Could you check a few things on this model? Use its own coordinates, in mm. A direction names the side the tool comes from. Give positions to 0.01 mm unless a question says otherwise; leave off trailing zeros. Loops run counter-clockwise (first coordinate to the right, second up) from the corner with the lowest first, then second, coordinate; pieces in that order, holes last. Notation, with made-up numbers: (69, -3.5) - (101, -3.5) arc R29 ccw to (101, 21.5) - close; hole circle Ø7 at (13.25, -28.5). An arc over 180 degrees is marked (long way). One line per item, written item: value. Start each with the question number.
Q1. I want a section at C-C (x = 99). Please give me the cut outline in (y, z).
Q2. I want a section at A-A (x = -55). Please give me the cut outline in (y, z), then the cut area to 3 significant figures.
Q3. For faces 1 (the face through (67, -2.54, 18)), 2 (the face through (-51, -2.54, 188)), 3 (the face through (-69, 0, 18)), which set-ups out of +Z, -Z, +X, -X, +Y, -Y let a thin tool reach every point of the face, with its end or its side?
Q4. I'm going to push flat-ended pins straight in: P1, Ø6, axis at x = -57.5, z = 176.5, coming from the +Y side; P2, Ø0.8, axis at x = 85.5, y = -1, coming from the +Z side; P3, Ø10, axis at x = 92.5, z = -11.5, coming from the -Y side. Where does each tip first touch, or does it pass through?
Q5. I want a section at B-B (z = 82.5). Please give me the cut outline in (x, y) (3 decimals).
Q6. If I drill on line 1 (Z direction, x = -32.5, y = -1); line 2 (Y direction, x = -67.5, z = -40.5); line 3 (Y direction, x = -7.5, z = 166.5), over which ranges is the centre line in solid material (lowest first)? Write a range as from..to.
```python
from build123d import *

# Parameters (mm, degrees)
F0_W     = 9.525
F0_H     = 381
F2_W     = 184.15
F2_H     = 127
F2_W_2   = 254
F2_H_2   = 190.5
F3_DEPTH = 2.54


with BuildPart() as f1:
    # F0 (on Front) → F1 (revolve)
    with BuildSketch(Plane.XZ):
        with Locations((4.7625, 60.951888)):
            Rectangle(F0_W, F0_H)
    revolve(axis=Axis((0, 0, 60.951888), (0, 0, 1)))

    # F2 (on Front) → F3 (join)
    with BuildSketch(Plane.XZ):
        with Locations((0, 187.531114)):
            Rectangle(F2_W, F2_H)
        with Locations((0, 16.501888)):
            Rectangle(F2_W_2, F2_H_2)
    extrude(amount=F3_DEPTH)


solid = f1.part
```
Worked answers:
1. outline: (-2.54, -78.75) - (0, -78.75) - (0, 111.75) - (-2.54, 111.75) - close
2. outline: (-2.54, -78.75) - (0, -78.75) - (0, 111.75) - (-2.54, 111.75) - close; (-2.54, 124.03) - (0, 124.03) - (0, 251.03) - (-2.54, 251.03) - close
2. area: 806 mm²
3. face 1: +Z, -Z, +X, -Y
3. face 2: +Z, -Z, -X, -Y
3. face 3: +Z, -Z, -X, +Y
4. P1: stops at y = 0
4. P2: stops at z = 251.03
4. P3: stops at y = -2.54
5. outline: (-127, -2.54) - (-9.18, -2.54) arc R9.525 ccw to (9.18, -2.54) - (127, -2.54) - (127, 0) - (9.525, 0) arc R9.525 ccw to (-9.525, 0) - (-127, 0) - close
6. line 1: z = -78.75..111.75, 124.03..251.03
6. line 2: y = -2.54..0
6. line 3: y = -5.87..5.87
